from build123d import *

# Parameters (mm, degrees)
SKETCH_R        = 1.75
PAD_DEPTH       = 25
SKETCH001_W     = 18
SKETCH001_H     = 3
POCKET_DEPTH    = 9.55
SKETCH002_W     = 5.8
SKETCH002_H     = 2
POCKET001_DEPTH = 9
SKETCH003_W     = 3.2
SKETCH003_H     = 2.3
SKETCH003_W_2   = 2.3
SKETCH003_H_2   = 3.2
POCKET002_DEPTH = 50.001
SKETCH004_R     = 1.75
PAD001_DEPTH    = 2
SKETCH005_R     = 1.75
PAD002_DEPTH    = 2
CHAMFER_SIZE    = 1.25


with BuildPart() as part:
    # Sketch → Pad (new body, symmetric)
    with BuildSketch(Plane.XY):
        Polygon((0, -4), (4, 0), (12, 0), (12, -8.5), (8.5, -12), (0, -12), align=None)
        with Locations((7, -7)):
            Circle(SKETCH_R, mode=Mode.SUBTRACT)
    extrude(amount=PAD_DEPTH, both=True)

    # Sketch001 (on Face4 of Pad) → Pocket (cut)
    with BuildSketch(Plane(origin=(10.25, -10.25, 0), x_dir=(0.707107, 0.707107, 0), z_dir=(0.707107, -0.707107, 0))):
        with Locations((0, 23.5)):
            Rectangle(SKETCH001_W, SKETCH001_H)
        with Locations((0, -23.5)):
            Rectangle(SKETCH001_W, SKETCH001_H)
    extrude(amount=-POCKET_DEPTH, mode=Mode.SUBTRACT)

    # Sketch002 (on Face12 of Pocket) → Pocket001 (cut)
    with BuildSketch(Plane(origin=(10.25, -10.25, 0), x_dir=(0.707107, 0.707107, 0), z_dir=(0.707107, -0.707107, 0))):
        with Locations((0, 17)):
            Rectangle(SKETCH002_W, SKETCH002_H)
        with Locations((0, -17)):
            Rectangle(SKETCH002_W, SKETCH002_H)
    extrude(amount=-POCKET001_DEPTH, mode=Mode.SUBTRACT)

    # Sketch003 (on Face4 of Pocket001) → Pocket002 (cut, through all)
    with BuildSketch(Plane(origin=(0, 0, -25), x_dir=(1, 0, 0), z_dir=(0, 0, -1))):
        with Locations((3.6, 10.85)):
            Rectangle(SKETCH003_W, SKETCH003_H)
        with Locations((10.85, 3.6)):
            Rectangle(SKETCH003_W_2, SKETCH003_H_2)
    extrude(amount=-POCKET002_DEPTH, mode=Mode.SUBTRACT)

    # Sketch004 (on Face2 of Pocket002) → Pad001 (join)
    with BuildSketch(Plane(origin=(0, 0, 0), x_dir=(0, -1, 0), z_dir=(-1, 0, 0))):
        with BuildLine():
            Line((12, 4), (15, 4))
            ThreePointArc((15, -4), (19, 0), (15, 4))
            Line((15, -4), (12, -4))
            Line((12, -4), (12, 4))
        make_face()
        with Locations((15, 0)):
            Circle(SKETCH004_R, mode=Mode.SUBTRACT)
    extrude(amount=-PAD001_DEPTH)

    # Sketch005 (on Face3 of Pad001) → Pad002 (join)
    with BuildSketch(Plane(origin=(0, 0, 0), x_dir=(-1, 0, 0), z_dir=(0, 1, 0))):
        with BuildLine():
            Line((-12, 4), (-15, 4))
            ThreePointArc((-15, 4), (-19, 0), (-15, -4))
            Line((-15, -4), (-12, -4))
            Line((-12, -4), (-12, 4))
        make_face()
        with Locations((-15, 0)):
            Circle(SKETCH005_R, mode=Mode.SUBTRACT)
    extrude(amount=-PAD002_DEPTH)

    # Chamfer
    chamfer_edges = [part.edges().sort_by_distance(p)[0] for p in [
        (16.75, 0, 0),
        (0, -13.25, 0),
    ]]
    chamfer(chamfer_edges, length=CHAMFER_SIZE)


solid = part.part
Model file for the job. Use its own axes, mm. A direction names the side the tool comes from. Round coordinates to 2 decimals unless told otherwise and drop trailing zeros. Order: outer loops, then holes, each group sorted by start corner. A loop starts at its lowest first (then second) coordinate and runs counter-clockwise, first axis right, second up.
(1) Pull direction Z, two halves, no side cores. Call faces 5 (the face through (5.2, -11, 0)), 6 (the face through (5, -6, -22)), 7 (the face through (7, -9, 16)): released by +Z, released by -Z, zero draft, split by the parting line, or undercut.
(2) Band-saw the part on A-A (z = 11). List the corners of the cut face in (x, y), then the cut area to 3 significant figures.
(3) Band-saw the part on C-C (x = 4.5). List the corners of the cut face in (y, z), then the cut area to 3 significant figures.
(4) Pin check, flat tips, straight feed: pin 1 (10 mm diameter, centred on y = -13, z = -16, fed in from +X); pin 2 (10 mm diameter, centred on x = 7.5, y = -14, fed in from -Z); pin 3 (1 mm diameter, centred on y = -3, z = 2, fed in from +X). Stop position of each tip, or through.
(5) Drill centre lines: line 1 (Z direction, x = 8.5, y = -5.25); line 2 (Y direction, x = 7, z = -20.05); line 3 (X direction, y = -7, z = -6.5). Where is each one in solid material? Low to high.
(6) Band-saw the part on B-B (x = 11.5). List the corners of the cut face in (y, z), then the cut area to 3 significant figures.
(7) 3-axis set-ups, long thin cutter, end or side, ignore diameter. For faces 1 (the face through (4, -9.7, 0)), 2 (the face through (1, -12, -13)), 3 (the face through (13, -1, 4)), 4 (the face through (9, -4.9, -17)): which of +Z, -Z, +X, -X, +Y, -Y reach the whole face in a straight line?
Verdict:
1. face 5: zero draft
1. face 6: released by -Z
1. face 7: undercut
2. outline: (0, -12) - (2, -12) - (2, -9.7) - (5.2, -9.7) - (5.2, -12) - (8.5, -12) - (12, -8.5) - (12, -5.2) - (9.7, -5.2) - (9.7, -2) - (12, -2) - (12, 0) - (4, 0) - (0, -4) - close; hole circle Ø3.5 at (7, -7)
2. area: 106 mm2
3. outline: (-9.7, -22) - (-2.49, -22) - (-2.49, -25) - (0, -25) - (0, 25) - (-2.49, 25) - (-2.49, 22) - (-9.7, 22) - close; hole (-8.6, -18) - (-3.27, -18) - (-3.27, -16) - (-8.6, -16) - close; hole (-8.6, 16) - (-3.27, 16) - (-3.27, 18) - (-8.6, 18) - close
3. area: 420 mm2
4. pin 1: stops at x = 12
4. pin 2: stops at z = -22
4. pin 3: stops at x = 9.7
5. line 1: z = -22 to -18, -16 to 16, 18 to 22
5. line 2: y = -12 to -8.75, -5.25 to 0
5. line 3: x = 0 to 5.25, 8.75 to 12
6. outline: (-9, -22) - (-5.2, -22) - (-5.2, 22) - (-9, 22) - (-9, 18) - (-7.4, 18) - (-7.4, 16) - (-9, 16) - (-9, -16) - (-7.4, -16) - (-7.4, -18) - (-9, -18) - close; (-2, -22) - (0, -22) - (0, 22) - (-2, 22) - close
6. area: 249 mm2
7. face 1: +Z, -Z, -Y
7. face 2: -Z, +X, -X, -Y
7. face 3: +Z, +X, +Y, -Y
7. face 4: none
